Could you check a few things on this model? Use its own coordinates, in mm. Face numbers are marked on the shaded views. A direction names the side the tool comes from. Round coordinates to 2 decimals unless told otherwise and drop trailing zeros. Loops run counter-clockwise (first coordinate to the right, second up) from the corner with the lowest first, then second, coordinate; pieces in that order, holes last. Notation, with made-up numbers: (71, 65.25) -> (117, 65.25) arc R25 cw to (117, 102.25) -> close; hole circle Ø1 at (-23, -27.5). An arc over 180 degrees is marked (long way). One line per item, written item: value.
from build123d import *

# Parameters (mm, degrees)
SKETCH1_W           = 1524
SKETCH1_H           = 355.6
BOSS_EXTRUDE1_DEPTH = 25.4
BOSS_EXTRUDE5_DEPTH = 25.4
BOSS_EXTRUDE6_DEPTH = 762
SKETCH7_R           = 76.2
CUT_EXTRUDE1_DEPTH  = 1575.8
SKETCH8_R           = 19.05
CUT_EXTRUDE2_DEPTH  = 1575.8


with BuildPart() as part:
    # Sketch1 → Boss-Extrude1 (new body)
    with BuildSketch(Plane.XY):
        with Locations((737.21023766, 170.176599634)):
            Rectangle(SKETCH1_W, SKETCH1_H)
    extrude(amount=BOSS_EXTRUDE1_DEPTH)

    # Sketch5 → Boss-Extrude5 (add)
    with BuildSketch(Plane.ZY.offset(24.78976234)):
        with BuildLine():
            Line((0, 347.976599634), (381, 347.976599634))
            Line((381, 347.976599634), (381, 141.861776851))
            ThreePointArc((381, 141.861776851), (303.930942088, 33.773491198), (177.8, -7.623400366))
            Line((177.8, -7.623400366), (0, -7.623400366))
            Line((0, -7.623400366), (0, 347.976599634))
        make_face()
    boss_extrude5 = extrude(amount=BOSS_EXTRUDE5_DEPTH)

    # Sketch6 → Boss-Extrude6 (add)
    with BuildSketch(Plane(origin=(-24.78976234, 0, 0), x_dir=(0, 0, -1), z_dir=(1, 0, 0))):
        Polygon((-25.4, 347.976599634), (-381, 347.976599634), (-381, 141.861776851), (-368.3, 141.861776851), (-368.3, 335.276599634), (-25.4, 335.276599634), align=None)
    boss_extrude6 = extrude(amount=BOSS_EXTRUDE6_DEPTH)

    # Mirror2: Boss-Extrude5, Boss-Extrude6 across plane
    add(boss_extrude5.mirror(Plane(origin=(737.21023766, 0, 0), x_dir=(0, 0, 1), z_dir=(1, 0, 0))))
    add(boss_extrude6.mirror(Plane(origin=(737.21023766, 0, 0), x_dir=(0, 0, 1), z_dir=(1, 0, 0))))

    # Sketch7 → Cut-Extrude1 (cut, through all)
    with BuildSketch(Plane.ZY.offset(50.18976234)):
        with Locations((203.2, 170.176599634)):
            Circle(SKETCH7_R)
    extrude(amount=-CUT_EXTRUDE1_DEPTH, mode=Mode.SUBTRACT)

    # Sketch8 → Cut-Extrude2 (cut, through all)
    with BuildSketch(Plane.ZY.offset(50.18976234)):
        with Locations((330.2, 129.161776851)):
            Circle(SKETCH8_R)
    extrude(amount=-CUT_EXTRUDE2_DEPTH, mode=Mode.SUBTRACT)


solid = part.part
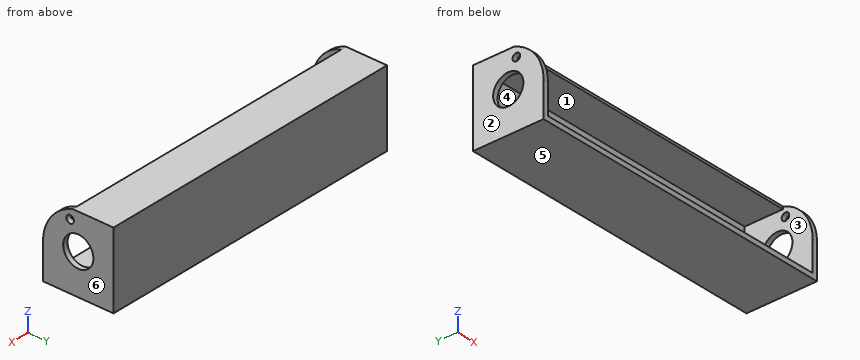
(1) Thinking about a two-plate mould opening in Z: for the marked faces 3, 4, 5 and 6, which applies, released by +Z, released by -Z, zero draft, split by the parting line, or undercut?
Recorded:
face 3: undercut
face 4: undercut
face 5: released by -Z
face 6: zero draft
(2) If we section it at B-B, the plane x = 1425: Please give me the cut outline in (y, z), then the cut area to 3 significant figures.
Recorded:
outline: (-7.62, 0) -> (347.98, 0) -> (347.98, 381) -> (141.86, 381) -> (141.86, 368.3) -> (335.28, 368.3) -> (335.28, 25.4) -> (-7.62, 25.4) -> close
area: 16,000 mm²
(3) If I drill on L1, parallel to X at y = 265.5, z = 217.5; L2, parallel to Z at x = 1426, y = 305.5; L3, parallel to Y at x = 572, z = 277, over which ranges is the centre line in solid material (lowest first)?
Recorded:
L1: -50.19 to -24.79, 1499.21 to 1524.61
L2: 0 to 25.4, 368.3 to 381
L3: 335.28 to 347.98
(4) If we section it at D-D, the plane z = 330.2: Please give me the cut outline in (x, y).
Recorded:
outline: (-50.19, 56.64) -> (-24.79, 56.64) -> (-24.79, 110.11) -> (-50.19, 110.11) -> close; (-50.19, 148.21) -> (-24.79, 148.21) -> (-24.79, 335.28) -> (1499.21, 335.28) -> (1499.21, 148.21) -> (1524.61, 148.21) -> (1524.61, 347.98) -> (-50.19, 347.98) -> close; (1499.21, 56.64) -> (1524.61, 56.64) -> (1524.61, 110.11) -> (1499.21, 110.11) -> close
(5) If we section it at C-C, the plane y = 64: Please give me the cut outline in (x, z), then the cut area to 3 significant figures.
Recorded:
outline: (-50.19, 0) -> (1524.61, 0) -> (1524.61, 337.05) -> (1499.21, 337.05) -> (1499.21, 25.4) -> (-24.79, 25.4) -> (-24.79, 337.05) -> (-50.19, 337.05) -> close
area: 55,800 mm²
(6) For the marked faces 1 and 2, which set-ups out of +Z, -Z, +X, -X, +Y, -Y let a thin tool reach every point of the face, with its end or its side?
Recorded:
face 1: -Y
face 2: +Z, -Z, -X, +Y, -Y
(7) I'm going to push flat-ended pins straight in: pin 1 Ø4 at (x, z) = (151, 49) entering from -Y; pin 2 Ø6.5 at (x, z) = (1058.5, 377.5) entering from -Y. Where does each tip first touch, or does it pass through?
Recorded:
pin 1: y = 335.28
pin 2: y = 141.86
(8) If we section it at A-A, the plane z = 164: Please give me the cut outline in (x, y).
Recorded:
outline: (-50.19, -7.62) -> (-24.79, -7.62) -> (-24.79, 104.83) -> (-50.19, 104.83) -> close; (-50.19, 235.52) -> (-24.79, 235.52) -> (-24.79, 335.28) -> (1499.21, 335.28) -> (1499.21, 235.52) -> (1524.61, 235.52) -> (1524.61, 347.98) -> (-50.19, 347.98) -> close; (1499.21, -7.62) -> (1524.61, -7.62) -> (1524.61, 104.83) -> (1499.21, 104.83) -> close
